Work out the finished part from the listing and answer in its coordinate system (mm). Give positions to 0.01 mm unless a question says otherwise; leave off trailing zeros. Loops run counter-clockwise (first coordinate to the right, second up) from the corner with the lowest first, then second, coordinate; pieces in that order, holes last. Notation, with made-up numbers: M -3.75,67.25 L 2.25,67.25 A20 ccw 2.25,105.25 Z; hole C 53,41.25 d8. An arc over 180 degrees is marked long. Write item = value, one per line. Start each with the question number.
1. Section B-B on z = 2 is taken. Give the number of separate pieces and of enclosed holes in the cut face, plus the area to 3 significant figures.
2. Section A-A on y = 44 is taken. Determine the outline of the cut face in (x, z).
3. Section C-C on x = -162.5 is taken. Determine the outline of the cut face in (y, z), plus the area to 4 significant figures.
4. Consider L1, parallel to X at y = 76, z = 1.25; L2, parallel to X at y = 47.5, z = 1.85; L3, parallel to Y at x = -225, z = 2. Determine where each line is inside the solid, lowest interval first. Write a range as [from, to].
5. The mould has two halves that part along X. Classify faces 1 (the face through (-229.77, 129, 1.97)), 2 (the face through (-4, -124, 4)): released by +X, released by -X, zero draft, split by the parting line, or undercut.
```python
from build123d import *

# Parameters (mm, degrees)
F0_W     = 480
F0_H     = 200
F1_DEPTH = 4
F3_D     = 10
F4_SIZE  = 0.5


with BuildPart() as f1:
    # F0 (on Top) → F1 (new body)
    with BuildSketch(Plane.XY):
        with BuildLine():
            Line((-274, -142), (274, -142))
            ThreePointArc((274, -142), (279.656854, -139.656854), (282, -134))
            Line((282, -134), (282, 134))
            ThreePointArc((282, 134), (279.656854, 139.656854), (274, 142))
            Line((274, 142), (-274, 142))
            ThreePointArc((-274, 142), (-279.656854, 139.656854), (-282, 134))
            Line((-282, 134), (-282, -134))
            ThreePointArc((-282, -134), (-279.656854, -139.656854), (-274, -142))
        make_face()
        Rectangle(F0_W, F0_H, mode=Mode.SUBTRACT)
    extrude(amount=F1_DEPTH)

    # F3 (through all)
    with Locations(Plane.XY.offset(4)):
        with Locations((-225, 127.5), (-75, 127.5), (75, 127.5), (225, 127.5), (265.5, 75), (265.5, -75), (225, -127.5), (75, -127.5), (-75, -127.5), (-225, -127.5), (-267.5, 75), (-267.5, -75)):
            Hole(F3_D / 2)

    # F4
    f4_edges = [f1.edges().sort_by_distance(p)[0] for p in [
        (0, -142, 4),
        (-274, -142, 2),
        (274, -142, 2),
        (0, -142, 0),
    ]]
    chamfer(f4_edges, length=F4_SIZE)


solid = f1.part
```
Verdict:
q1.separate_pieces = 1
q1.enclosed_holes = 13
q1.area = 63,200 mm2
q2.outline = M -282,0.5 L -281.5,0 L -240,0 L -240,4 L -281.5,4 L -282,3.5 Z; M 240,0 L 281.5,0 L 282,0.5 L 282,3.5 L 281.5,4 L 240,4 Z
q3.outline = M -142,0.5 L -141.5,0 L -100,0 L -100,4 L -141.5,4 L -142,3.5 Z; M 100,0 L 141.5,0 L 142,0.5 L 142,3.5 L 141.5,4 L 100,4 Z
q3.area = 335.5 mm2
q4.L1 = [-282, -272.4], [-262.6, -240], [240, 260.6], [270.4, 282]
q4.L2 = [-282, -240], [240, 282]
q4.L3 = [-142, -132.5], [-122.5, -100], [100, 122.5], [132.5, 142]
q5.face_1 = undercut
q5.face_2 = zero draft
